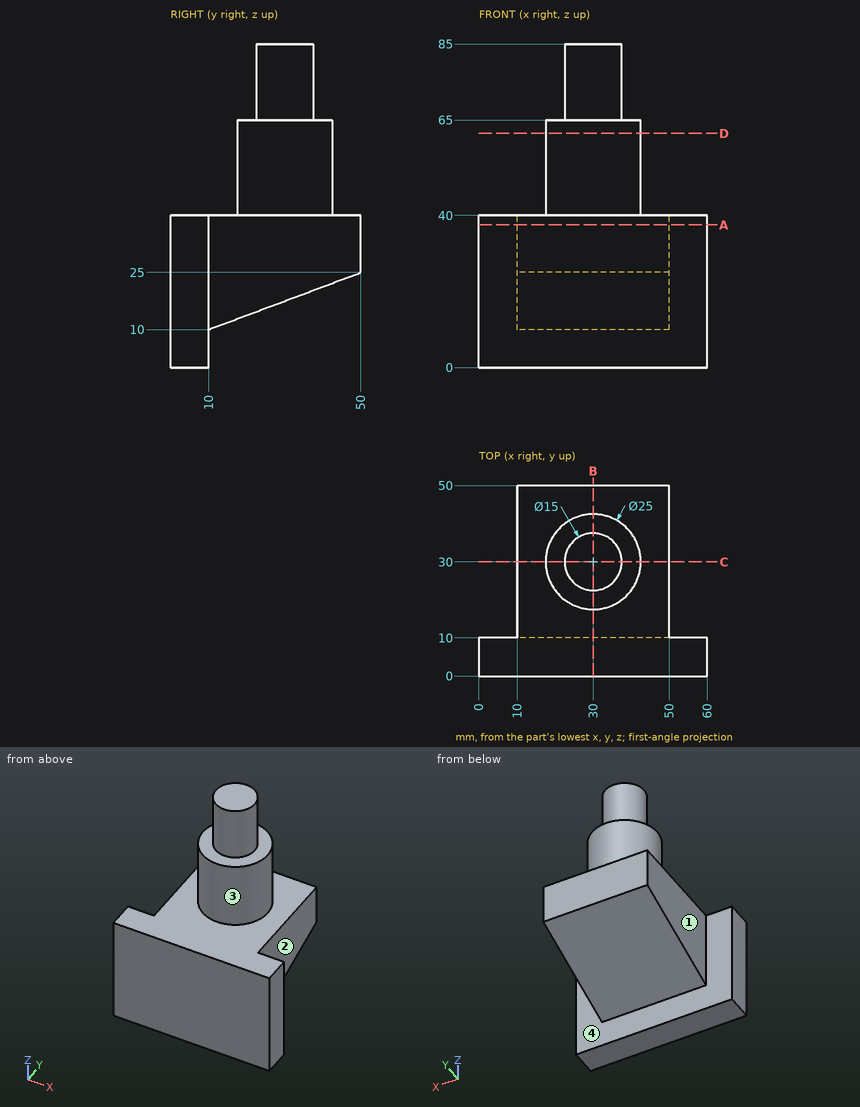
For this review, use the dimensioned drawing (mm, ordinates from the lowest corner) and the shaded views. A direction names the side the tool comes from. Coordinates: 2 decimals unless noted, no trailing zeros. Loops run counter-clockwise (first coordinate to the right, second up) from the corner with the lowest first, then second, coordinate; pieces in that order, holes last. Notation, with made-up numbers: (55.5, 34.5) - (61.5, 34.5) arc R21 cw to (61.5, 40.5) - close; hole circle Ø2 at (8, -7). An arc over 180 degrees is marked (long way). Use one line per item in the form item = value. Start each with the question number.
1) For pin 1 (2 mm diameter, centred on y = 12.5, z = 31.5, fed in from +X); pin 2 (12 mm diameter, centred on y = 33.5, z = 22, fed in from -X); pin 3 (1 mm diameter, centred on x = 8, z = 11, fed in from +Y), all flat-tipped, find the tip position at first contact; note any pin that passes through.
2) For the marked faces 1, 2, 3 and 4, list the 3-axis set-ups (+Z, -Z, +X, -X, +Y, -Y) from which the entire face can be reached by the end or side of a thin tool; tool diameter is ignored.
3) Take a section at A-A (z = 37.5). State the section outline as (x, y) points.
4) Take a section at D-D (z = 61.5). State the section outline as (x, y) points.
5) Take a section at C-C (y = 30). State the section outline as (x, z) points, plus the area to 4 significant figures.
6) Take a section at B-B (x = 30). State the section outline as (y, z) points, plus the area to 4 significant figures.
7) To check wall thickness, follow probe 1 along Z at (x, y) = (25, 7.5); probe 2 along X at (y, z) = (11.5, 38.5); probe 3 along Y at (x, z) = (26, 4). State the ranges of each line that lie inside material, in increasing order. Write a range as from..to.
From the geometry:
q1.pin_1 = 50
q1.pin_2 = 10
q1.pin_3 = 10
q2.face_1 = +Z, -Z, -X, +Y
q2.face_2 = +Z, -Z, +X, +Y
q2.face_3 = +Z
q2.face_4 = -Z, +Y
q3.outline = (0, 0) - (60, 0) - (60, 10) - (50, 10) - (50, 50) - (10, 50) - (10, 10) - (0, 10) - close
q4.outline = circle Ø25 at (30, 30)
q5.outline = (10, 17.5) - (50, 17.5) - (50, 40) - (42.5, 40) - (42.5, 65) - (37.5, 65) - (37.5, 85) - (22.5, 85) - (22.5, 65) - (17.5, 65) - (17.5, 40) - (10, 40) - close
q5.area = 1,825 mm2
q6.outline = (0, 0) - (10, 0) - (10, 10) - (50, 25) - (50, 40) - (42.5, 40) - (42.5, 65) - (37.5, 65) - (37.5, 85) - (22.5, 85) - (22.5, 65) - (17.5, 65) - (17.5, 40) - (0, 40) - close
q6.area = 2,225 mm2
q7.probe_1 = 0..40
q7.probe_2 = 10..50
q7.probe_3 = 0..10
